from build123d import *

# Parameters (mm, degrees)
SKETCH1_W           = 6.35
SKETCH1_H           = 76.2
BOSS_EXTRUDE1_DEPTH = 63.5
SKETCH2_W           = 6.35
SKETCH2_H           = 12.7
BOSS_EXTRUDE2_DEPTH = 6.35
SKETCH3_W           = 50.8
SKETCH3_H           = 6.35
CUT_EXTRUDE1_DEPTH  = 80.818262321


with BuildPart() as part:
    # Sketch1 → Boss-Extrude1 (new body)
    with BuildSketch(Plane.XY):
        with Locations((111.125, 0)):
            Rectangle(SKETCH1_W, SKETCH1_H)
    extrude(amount=BOSS_EXTRUDE1_DEPTH)

    # Sketch2 → Boss-Extrude2 (add)
    with BuildSketch(Plane(origin=(114.3, 0, 0), x_dir=(0, 0, -1), z_dir=(1, 0, 0))):
        with Locations((-66.675, -31.75)):
            Rectangle(SKETCH2_W, SKETCH2_H)
        with Locations((-66.675, 31.75)):
            Rectangle(SKETCH2_W, SKETCH2_H)
        with Locations((3.175, 31.75)):
            Rectangle(SKETCH2_W, SKETCH2_H)
        with Locations((3.175, -31.75)):
            Rectangle(SKETCH2_W, SKETCH2_H)
    extrude(amount=-BOSS_EXTRUDE2_DEPTH)

    # Sketch3 → Cut-Extrude1 (cut, through all)
    with BuildSketch(Plane(origin=(114.3, 0, 0), x_dir=(0, 0, -1), z_dir=(1, 0, 0))):
        with Locations((-31.75, 31.75)):
            Rectangle(SKETCH3_W, SKETCH3_H)
        with Locations((-31.75, -34.925)):
            Rectangle(SKETCH3_W, SKETCH3_H)
    extrude(amount=-CUT_EXTRUDE1_DEPTH, mode=Mode.SUBTRACT)


solid = part.part
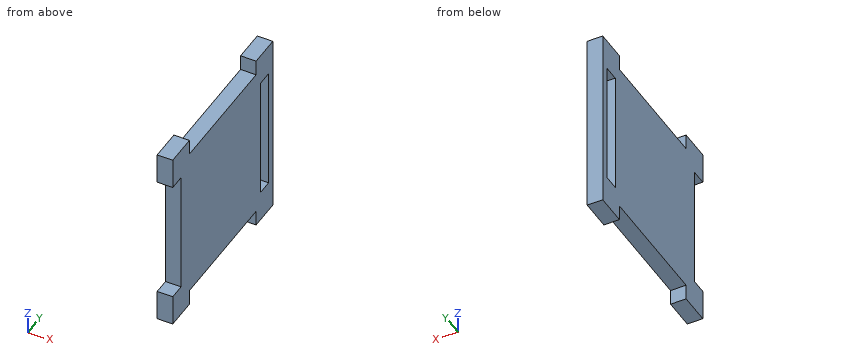
The listing builds one solid part. Answer for the finished solid, in the listing's coordinates (mm). Round coordinates to 2 decimals unless told otherwise and drop trailing zeros. Order: outer loops, then holes, each group sorted by start corner. A loop starts at its lowest first (then second) coordinate and runs counter-clockwise, first axis right, second up. Notation, with made-up numbers: M 3.5,64 L 21.5,64 A22 ccw 21.5,84 Z; hole C -25,39.5 d5. An arc over 180 degrees is marked long. Answer in a Markdown table with one row per item. Add a question column.
1) The part is cut by section A-A on z = 46.5. Determine the outline of the cut face in (x, y) (3 decimals), plus the area to 3 significant figures.
2) The part is cut by section C-C on y = -19. Determine the outline of the cut face in (x, z).
3) Flat-ended cylindrical pins translate along their axes: pin 1 Ø1.9 at (x, y) = (112, -12) entering from +Z; pin 2 Ø3 at (x, z) = (111.5, 23) entering from -Y. Find the tip coordinate at first contact, or state that the pin passes through.
4) The part is cut by section B-B on x = 112. Determine the outline of the cut face in (y, z) (3 decimals).
5) Consider line 1 along Y through (x, z) = (111.5, 39) (3 decimals); line 2 along Z through (x, y) = (111.75, 32); line 3 along Y through (x, z) = (114.25, 64.5). Determine where each line is inside the solid, lowest interval first. Write a range as from..to.
Findings below:
| question | item | result |
|---|---|---|
| 1 | outline | M 107.95,-31.75 L 114.3,-31.75 L 114.3,28.575 L 107.95,28.575 Z; M 107.95,34.925 L 114.3,34.925 L 114.3,38.1 L 107.95,38.1 Z |
| 1 | area | 403 mm² |
| 2 | outline | M 107.95,0 L 114.3,0 L 114.3,63.5 L 107.95,63.5 Z |
| 3 | pin 1 | stops at z = 63.5 |
| 3 | pin 2 | stops at y = -31.75 |
| 4 | outline | M -38.1,-6.35 L -25.4,-6.35 L -25.4,0 L 25.4,0 L 25.4,-6.35 L 38.1,-6.35 L 38.1,69.85 L 25.4,69.85 L 25.4,63.5 L -25.4,63.5 L -25.4,69.85 L -38.1,69.85 L -38.1,57.15 L -31.75,57.15 L -31.75,6.35 L -38.1,6.35 Z; hole M 28.575,6.35 L 34.925,6.35 L 34.925,57.15 L 28.575,57.15 Z |
| 5 | line 1 | y = -31.75..28.575, 34.925..38.1 |
| 5 | line 2 | z = -6.35..6.35, 57.15..69.85 |
| 5 | line 3 | y = -38.1..-25.4, 25.4..38.1 |
